For this review, take the finished solid that the model builds, in its own axes (mm). Face numbers are marked on the shaded views. A direction names the side the tool comes from. Round coordinates to 2 decimals unless told otherwise and drop trailing zeros. Loops run counter-clockwise (first coordinate to the right, second up) from the corner with the lowest first, then second, coordinate; pieces in that order, holes last.
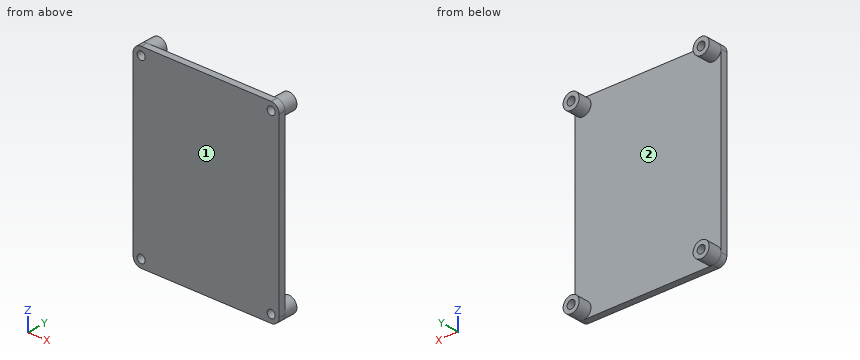
```python
from build123d import *

# Parameters (mm, degrees)
SKETCH1_W           = 54.5
SKETCH1_H           = 71
BOSS_EXTRUDE1_DEPTH = 2.5
SKETCH2_R           = 3
BOSS_EXTRUDE2_DEPTH = 5
FILLET1_R           = 3
SKETCH3_R           = 1.5
CUT_EXTRUDE1_DEPTH  = 7.5


with BuildPart() as part:
    # Sketch1 → Boss-Extrude1 (new body)
    with BuildSketch(Plane(origin=(0, 0, 0), x_dir=(1, 0, 0), z_dir=(0, 1, 0))):
        with Locations((-42.847381712, -51.275024631)):
            Rectangle(SKETCH1_W, SKETCH1_H)
    extrude(amount=BOSS_EXTRUDE1_DEPTH)

    # Sketch2 → Boss-Extrude2 (add)
    with BuildSketch(Plane(origin=(0, 2.5, 0), x_dir=(1, 0, 0), z_dir=(0, 1, 0))):
        with Locations(Location((-67.097381712, -18.775024631, 0), (0, 0, 90))):
            Circle(SKETCH2_R)
        with Locations(Location((-18.597381712, -18.775024631, 0), (0, 0, 90))):
            Circle(SKETCH2_R)
        with Locations(Location((-18.597381712, -83.775024631, 0), (0, 0, 270))):
            Circle(SKETCH2_R)
        with Locations(Location((-67.097381712, -83.775024631, 0), (0, 0, 270))):
            Circle(SKETCH2_R)
    extrude(amount=BOSS_EXTRUDE2_DEPTH)

    # Fillet1
    fillet1_edges = [part.edges().sort_by_distance(p)[0] for p in [
        (-70.097381712, 1.25, 15.775024631),
        (-15.597381712, 1.25, 15.775024631),
        (-15.597381712, 1.25, 86.775024631),
        (-70.097381712, 1.25, 86.775024631),
    ]]
    fillet(fillet1_edges, radius=FILLET1_R - 0.0001)  # a hair under: the kernel refuses the full size

    # Sketch3 → Cut-Extrude1 (cut)
    with BuildSketch(Plane(origin=(0, 7.5, 0), x_dir=(1, 0, 0), z_dir=(0, 1, 0))):
        with Locations(Location((-67.097381712, -18.775024631, 0), (0, 0, 270))):
            Circle(SKETCH3_R)
        with Locations(Location((-18.597381712, -18.775024631, 0), (0, 0, 270))):
            Circle(SKETCH3_R)
        with Locations(Location((-18.597381712, -83.775024631, 0), (0, 0, 270))):
            Circle(SKETCH3_R)
        with Locations(Location((-67.097381712, -83.775024631, 0), (0, 0, 270))):
            Circle(SKETCH3_R)
    extrude(amount=-CUT_EXTRUDE1_DEPTH, mode=Mode.SUBTRACT)


solid = part.part
```
(1) Add section A-A (y = 4.25). Give the boundary of the cut face in (x, z), plus the area to 3 significant figures.
(2) For the marked faces 1 and 2, list the 3-axis set-ups (+Z, -Z, +X, -X, +Y, -Y) from which the entire face can be reached by the end or side of a thin tool; tool diameter is ignored.
(3) Add section B-B (x = -52). Give the boundary of the cut face in (y, z).
(4) Add section C-C (z = 24). Give the boundary of the cut face in (x, y).
(5) For L1, parallel to Y at x = -50, z = 73, list the stretches that pass through material, from the lowest coordinate up.
(6) Insertion check: pin 1 Ø12 at (x, z) = (-23, 54.5) entering from +Y; pin 2 Ø3.5 at (x, z) = (-18.6, 18.78) entering from -Y. Each pin has a flat end and moves straight along its axis. Give the tip position at first contact, or say it passes through.
Outcome:
1. outline: circle Ø6 at (-67.1, 18.78); circle Ø6 at (-67.1, 83.78); circle Ø6 at (-18.6, 18.78); circle Ø6 at (-18.6, 83.78); hole circle Ø3 at (-67.1, 18.78); hole circle Ø3 at (-67.1, 83.78); hole circle Ø3 at (-18.6, 18.78); hole circle Ø3 at (-18.6, 83.78)
1. area: 84.8 mm2
2. face 1: +Z, -Z, +X, -X, -Y
2. face 2: +Y
3. outline: (0, 15.78) - (2.5, 15.78) - (2.5, 86.78) - (0, 86.78) - close
4. outline: (-70.1, 0) - (-15.6, 0) - (-15.6, 2.5) - (-70.1, 2.5) - close
5. L1: y = 0 to 2.5
6. pin 1: stops at y = 2.5
6. pin 2: stops at y = 0
